Design review of the part built by this model. Coordinates are the model's own, in mm. A direction names the side the tool comes from. Coordinates: 2 decimals unless noted, no trailing zeros. Write each loop counter-clockwise with the first axis right and the second up, starting at its lowest first coordinate (ties: lowest second). Pieces come first, ordered by that corner, then holes. Notation, with made-up numbers: (-33.5, 8) -> (-20.5, 8) arc R28 cw to (-20.5, 33) -> close; hole circle Ø7 at (-31.5, 41.25). An arc over 180 degrees is marked (long way). Answer in a Markdown table with one row per item. Add a question column.
Item 1: Take a section at B-B, the plane z = 7.5. Write out the cut boundary in (x, y), and give its area (3 significant figures).
Item 2: Take a section at D-D, the plane x = -40. Write out the cut boundary in (y, z).
Item 3: Take a section at C-C, the plane x = 0. Write out the cut boundary in (y, z).
Item 4: To check wall thickness, follow line 1 (Y direction, x = 0, z = 23); line 2 (Z direction, x = 59, y = -22.5); line 3 (X direction, y = -2, z = 41). State the ranges of each line that lie inside material, in increasing order.
Item 5: Draft analysis for pull direction Y (two halves, no side actions). For faces 3 (the face through (-50, 0, 65)), 4 (the face through (-1, -30, 27)), 5 (the face through (-2.2, -9.89, 30.42)), state which applies: released by +Y, released by -Y, zero draft, split by the parting line, or undercut.
Item 6: Take a section at A-A, the plane y = 0. Write out the cut boundary in (x, z), and give its area (3 significant figures).
Item 7: For faces 1 (the face through (35, 0, 70)), 2 (the face through (24.634, 0.458, 64.93)), list the 3-axis set-ups (+Z, -Z, +X, -X, +Y, -Y) from which the entire face can be reached by the end or side of a thin tool; tool diameter is ignored.
from build123d import *

# Parameters (mm, degrees)
F0_W     = 140
F0_H     = 60
F1_DEPTH = 60
F2_R     = 10
F5_DEPTH = 10
F4_R     = 10.13292
F6_DEPTH = 175
F3_R     = 10.418287
F7_DEPTH = 10
F8_R     = 5


with BuildPart() as f1:
    # F0 (on Top) → F1 (new body)
    with BuildSketch(Plane.XY):
        Rectangle(F0_W, F0_H)
    extrude(amount=F1_DEPTH)

    # F2 (on face) → F5 (join)
    with BuildSketch(Plane.XY.offset(60)):
        with Locations((-40, 0)):
            Circle(F2_R)
    extrude(amount=F5_DEPTH)

    # F4 (on face) → F6 (cut)
    with BuildSketch(Plane.XY.offset(60)):
        Circle(F4_R)
    extrude(amount=-F6_DEPTH, mode=Mode.SUBTRACT)

    # F3 (on face) → F7 (join)
    with BuildSketch(Plane.XY.offset(60)):
        with Locations((35.042234, 0)):
            Circle(F3_R)
    extrude(amount=F7_DEPTH)

    # F8
    f8_edges = [f1.edges().sort_by_distance(p)[0] for p in [
        (0, 30, 60),
        (70, 0, 60),
        (0, -30, 60),
        (-70, 0, 60),
        (-70, 30, 30),
        (-70, -30, 30),
        (70, -30, 30),
        (70, 30, 30),
    ]]
    fillet(f8_edges, radius=F8_R)


solid = f1.part
Answers:
| question | item | result |
|---|---|---|
| 1 | outline | (-70, -25) arc R5 ccw to (-65, -30) -> (65, -30) arc R5 ccw to (70, -25) -> (70, 25) arc R5 ccw to (65, 30) -> (-65, 30) arc R5 ccw to (-70, 25) -> close; hole circle Ø20.27 at (0, 0) |
| 1 | area | 8,060 mm^2 |
| 2 | outline | (-30, 0) -> (30, 0) -> (30, 55) arc R5 ccw to (25, 60) -> (10, 60) -> (10, 70) -> (-10, 70) -> (-10, 60) -> (-25, 60) arc R5 ccw to (-30, 55) -> close |
| 3 | outline | (-30, 0) -> (-10.13, 0) -> (-10.13, 60) -> (-25, 60) arc R5 ccw to (-30, 55) -> close; (10.13, 0) -> (30, 0) -> (30, 55) arc R5 ccw to (25, 60) -> (10.13, 60) -> close |
| 4 | line 1 | y = -30 to -10.13, 10.13 to 30 |
| 4 | line 2 | z = 0 to 60 |
| 4 | line 3 | x = -70 to -9.93, 9.93 to 70 |
| 5 | face 3 | split by the parting line |
| 5 | face 4 | released by -Y |
| 5 | face 5 | undercut |
| 6 | outline | (-70, 0) -> (-10.13, 0) -> (-10.13, 60) -> (-30, 60) -> (-30, 70) -> (-50, 70) -> (-50, 60) -> (-65, 60) arc R5 ccw to (-70, 55) -> close; (10.13, 0) -> (70, 0) -> (70, 55) arc R5 ccw to (65, 60) -> (45.46, 60) -> (45.46, 70) -> (24.62, 70) -> (24.62, 60) -> (10.13, 60) -> close |
| 6 | area | 7,580 mm^2 |
| 7 | face 1 | +Z, +X, -X, +Y, -Y |
| 7 | face 2 | +Z |
